Autodesk Inventor part; units mm, degrees
ref_plane "YZ Plane" through (0, 0, 0) normal (1, 0, 0) x (0, 1, 0)
ref_plane "XZ Plane" through (0, 0, 0) normal (0, 1, 0) x (-1, 0, 0)
ref_plane "XY Plane" through (0, 0, 0) normal (0, 0, 1) x (1, 0, 0)
sketch "Sketch1" plane through (0, 0, 0) normal (0, 1, 0) x (-1, 0, 0)
  circle A0 centre (0, 0) radius 3
  dimension "d0" = 6
extrude "Extrusion1" add sketch "Sketch1" along normal blind 6
sketch "Sketch2" plane through (0, 6, 0) normal (0, 1, 0) x (1, 0, 0)
  line L0 (-4.0415, 0) -> (-2.0207, 3.5)
  line L1 (-2.0207, 3.5) -> (2.0207, 3.5)
  line L2 (2.0207, 3.5) -> (4.0415, 0)
  line L3 (4.0415, 0) -> (2.0207, -3.5)
  line L4 (2.0207, -3.5) -> (-2.0207, -3.5)
  line L5 (-2.0207, -3.5) -> (-4.0415, 0)
  point P0 (0, 0)
  point P1 (0, 0)
  dimension "d3" = 7
extrude "Extrusion2" add sketch "Sketch2" along normal blind 3
sketch "Sketch3" plane through (0, 9, 0) normal (0, 1, 0) x (1, 0, 0)
  circle A0 centre (0, 0) radius 2.5
  dimension "d6" = 5
extrude "Extrusion3" add sketch "Sketch3" along normal blind 2
chamfer "Chamfer1" distance 2 angle 45 1 edges at (-2.5, 11, 0)
sketch "Sketch4" plane through (0, 0, 0) normal (0, -1, 0) x (1, 0, 0)
  circle A0 centre (0, 0) radius 0.5
hole "Hole1" at (0, 0, 0) direction (0, 1, 0) diameter 0.3 end through all countersink diameter 4 countersink angle 20
thread "Thread1"
properties part number "Chimera Nozzle" material "Brass"
Could you check a few things on this model? Use its own coordinates, in mm. A direction names the side the tool comes from. Coordinates: 2 decimals unless noted, no trailing zeros. Order: outer loops, then holes, each group sorted by start corner. A loop starts at its lowest first (then second) coordinate and runs counter-clockwise, first axis right, second up. Notation, with made-up numbers: M 8,66 L 26,66 A34 cw 26,98 Z; hole C 22,16 d8. An arc over 180 degrees is marked long. Use a Markdown table: item, result. Add a question column.
Q1. Which directions (+Z, -Z, +X, -X, +Y, -Y) give clear straight access to the entire face, cutting with the end or side of a thin tool? Please do faces 1 (the flat face through (3, 9, 0)), 2 (the flat face through (3, 7.5, -1.8)), 3 (the flat face through (-1, 6, -3)).
Q2. I want a section at B-B on z = 3.25. List the corners of the cut face in (x, y) for me.
Q3. I want a section at C-C on x = 3.25. List the corners of the cut face in (y, z) for me.
Q4. If I drill on L1, parallel to Y at x = -3.25, z = -0.5; L2, parallel to Z at x = 0, y = 1; L3, parallel to Z at x = 0.75, y = 3, over which ranges is the centre line in solid material (lowest first)?
Q5. We'd pull the mould along Z, two halves only. Please class faces 4 (the conical face through (-1.06, 5.17, 0.24)), 5 (the cylindrical face through (3, 3, 0)), 6 (the flat face through (-3.045, 7.479, -1.726)): pulls with the +Z half, pulls with the -Z half, needs draft (parallel to the pull), parting line crosses it, or undercut.
Q6. I'm going to push flat-ended pins straight in: pin 1 (4 mm diameter, centred on y = 7.5, z = 2.5, fed in from -X); pin 2 (1.5 mm diameter, centred on y = 7.5, z = 2, fed in from -X). Where does each tip first touch, or does it pass through?
Checked values:
| question | item | result |
|---|---|---|
| 1 | face 1 | +Y |
| 1 | face 2 | -Z, +X, +Y, -Y |
| 1 | face 3 | -Y |
| 2 | outline | M -2.17,6 L 2.17,6 L 2.17,9 L -2.17,9 Z |
| 3 | outline | M 6,-1.37 L 9,-1.37 L 9,1.37 L 6,1.37 Z |
| 4 | L1 | 6 to 9 |
| 4 | L2 | -3 to -1.82, 1.82 to 3 |
| 4 | L3 | -2.9 to -1.27, 1.27 to 2.9 |
| 5 | face 4 | undercut |
| 5 | face 5 | parting line crosses it |
| 5 | face 6 | pulls with the -Z half |
| 6 | pin 1 | x = -3.75 |
| 6 | pin 2 | x = -3.32 |
